Verification items for the finished model (mm, model axes). Round coordinates to 2 decimals unless told otherwise and drop trailing zeros. Loops run counter-clockwise (first coordinate to the right, second up) from the corner with the lowest first, then second, coordinate; pieces in that order, holes last. Notation, with made-up numbers: M 37.5,1.25 L 63.5,1.25 A22 ccw 63.5,39.25 Z; hole C -27,71 d9. An arc over 180 degrees is marked long. One line per item, written item: value.
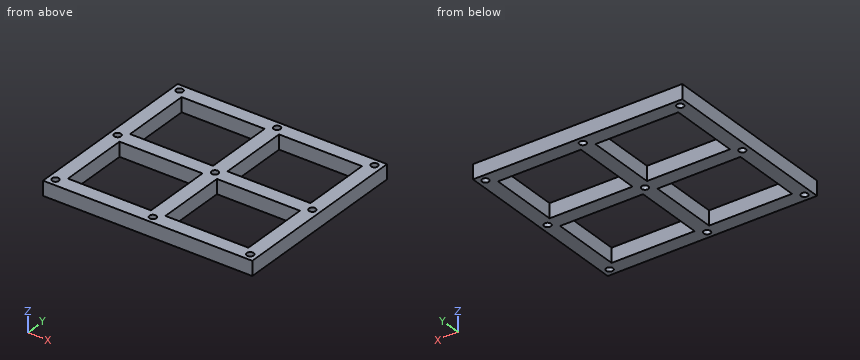
from build123d import *

# Parameters (mm, degrees)
F0_W     = 92
F0_H     = 81.05
F1_DEPTH = 6.35
F3_W     = 36.475
F3_H     = 31
F4_DEPTH = 6.35
F5_D     = 3


with BuildPart() as f1:
    # F0 (on Top) → F1 (new body)
    with BuildSketch(Plane.XY):
        Rectangle(F0_W, F0_H)
    extrude(amount=F1_DEPTH)

    # F3 (on face) → F4 (cut)
    with BuildSketch(Plane(origin=(0, 0, 0), x_dir=(1, 0, 0), z_dir=(0, 0, -1))):
        with Locations((-21.4125, 18.675)):
            Rectangle(F3_W, F3_H)
        with Locations((-21.4125, -18.675)):
            Rectangle(F3_W, F3_H)
        with Locations((21.4125, 18.675)):
            Rectangle(F3_W, F3_H)
        with Locations((21.4125, -18.675)):
            Rectangle(F3_W, F3_H)
    extrude(amount=-F4_DEPTH, mode=Mode.SUBTRACT)

    # F5 (through all)
    with Locations(Plane.XY.offset(6.35)):
        with Locations((-42.825, 37.35), (0, 37.35), (42.825, 37.35), (-42.825, 0), (0, 0), (42.825, 0), (-42.825, -37.35), (0, -37.35), (42.825, -37.35)):
            Hole(F5_D / 2)


solid = f1.part
(1) Sectioned sample at B-B on y = 0. Enter the section's corners in (x, z) (3 decimals), and give its area (3 significant figures).
Completed:
outline: M -46,0 L -44.325,0 L -44.325,6.35 L -46,6.35 Z; M -41.325,0 L -1.5,0 L -1.5,6.35 L -41.325,6.35 Z; M 1.5,0 L 41.325,0 L 41.325,6.35 L 1.5,6.35 Z; M 44.325,0 L 46,0 L 46,6.35 L 44.325,6.35 Z
area: 527 mm^2
(2) Sectioned sample at C-C on y = -20.5. Enter the section's corners in (x, z) (3 decimals), and give its area (3 significant figures).
Completed:
outline: M -46,0 L -39.65,0 L -39.65,6.35 L -46,6.35 Z; M -3.175,0 L 3.175,0 L 3.175,6.35 L -3.175,6.35 Z; M 39.65,0 L 46,0 L 46,6.35 L 39.65,6.35 Z
area: 121 mm^2
(3) Sectioned sample at A-A on x = -35.5. Enter the section's corners in (y, z) (3 decimals).
Completed:
outline: M -40.525,0 L -34.175,0 L -34.175,6.35 L -40.525,6.35 Z; M -3.175,0 L 3.175,0 L 3.175,6.35 L -3.175,6.35 Z; M 34.175,0 L 40.525,0 L 40.525,6.35 L 34.175,6.35 Z
(4) Sectioned sample at D-D on x = 0. Enter the section's corners in (y, z) (3 decimals), and give its area (3 significant figures).
Completed:
outline: M -40.525,0 L -38.85,0 L -38.85,6.35 L -40.525,6.35 Z; M -35.85,0 L -1.5,0 L -1.5,6.35 L -35.85,6.35 Z; M 1.5,0 L 35.85,0 L 35.85,6.35 L 1.5,6.35 Z; M 38.85,0 L 40.525,0 L 40.525,6.35 L 38.85,6.35 Z
area: 458 mm^2
(5) Depth check by flat-ended pin: pin 1 Ø2.5 at (x, y) = (-42.825, 37.35) entering from +Z; pin 2 Ø3.5 at (x, y) = (42.825, 0) entering from +Z. Enter the tip coordinate at first touch or a pass-through.
Completed:
pin 1: passes through
pin 2: stops at z = 6.35
(6) Thickness scan on L1, parallel to X at y = -19.5, z = 3 (3 decimals); L2, parallel to Y at x = -15.5, z = 2.25 (3 decimals); L3, parallel to Y at x = -1, z = 5.25 (3 decimals). Record the ranges inside material, lowest first. Write a range as from..to.
Completed:
L1: x = -46..-39.65, -3.175..3.175, 39.65..46
L2: y = -40.525..-34.175, -3.175..3.175, 34.175..40.525
L3: y = -40.525..-38.468, -36.232..-1.118, 1.118..36.232, 38.468..40.525
